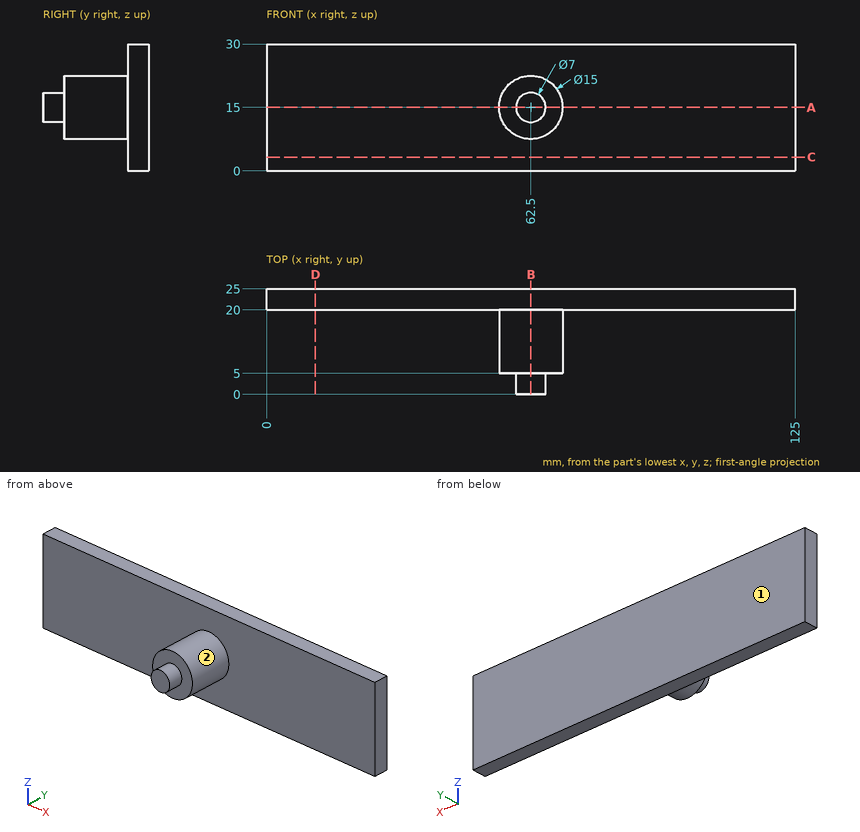
Source: three-view drawing plus pictorial views. Frame: mm from the lowest corner of the part. A direction names the side the tool comes from. Round coordinates to 2 decimals unless told otherwise and drop trailing zeros. Write each loop counter-clockwise with the first axis right and the second up, starting at its lowest first coordinate (ties: lowest second). Pieces come first, ordered by that corner, then holes. Notation, with made-up numbers: M -12.5,-23.5 L 0.5,-23.5 A11 ccw 0.5,-10.5 Z; hole C 60,32 d5. An arc over 180 degrees is marked long. Write each question's results on one line, items separated by ' | '.
Q1. Section query D-D (x = 11.5). Return loops of the section in (y, z).
Results:
outline: M 20,0 L 25,0 L 25,30 L 20,30 Z
Q2. Access query for the marked faces 1 and 2. Directions: +Z, -Z, +X, -X, +Y, -Y. A direction counts if a zero-diameter tool reaches every point of the face in a straight line with its end or side. Return the directions, or none.
Results:
face 1: +Z, -Z, +X, -X, +Y | face 2: -Y
Q3. Section query B-B (x = 62.5). Return loops of the section in (y, z), and give its area (3 significant figures).
Results:
outline: M 0,11.5 L 5,11.5 L 5,7.5 L 20,7.5 L 20,0 L 25,0 L 25,30 L 20,30 L 20,22.5 L 5,22.5 L 5,18.5 L 0,18.5 Z | area: 410 mm^2
Q4. Section query A-A (z = 15). Return loops of the section in (x, y), and give its area (3 significant figures).
Results:
outline: M 0,20 L 55,20 L 55,5 L 59,5 L 59,0 L 66,0 L 66,5 L 70,5 L 70,20 L 125,20 L 125,25 L 0,25 Z | area: 885 mm^2
Q5. Section query C-C (z = 3.25). Return loops of the section in (x, y), and give its area (3 significant figures).
Results:
outline: M 0,20 L 125,20 L 125,25 L 0,25 Z | area: 625 mm^2
Q6. Line query: line 1 along Y through (x, z) = (75, 16); line 2 along X through (y, z) = (8.25, 17.5); line 3 along Z through (x, y) = (65, 13.75). Output: solid intervals per line, ascending.
Results:
line 1: y = 20 to 25 | line 2: x = 55.43 to 69.57 | line 3: z = 7.93 to 22.07
Q7. Pin query (flat end, axial travel): P1, Ø6, axis at x = 61, z = 23, coming from the -Y side; P2, Ø15, axis at x = 93.5, z = 9.5, coming from the -Y side; P3, Ø1.5, axis at y = 15.5, z = 17.5, coming from the +X side. Return the tip coordinate at first contact, or that it passes through.
Results:
P1: stops at y = 5 | P2: stops at y = 20 | P3: stops at x = 69.79
